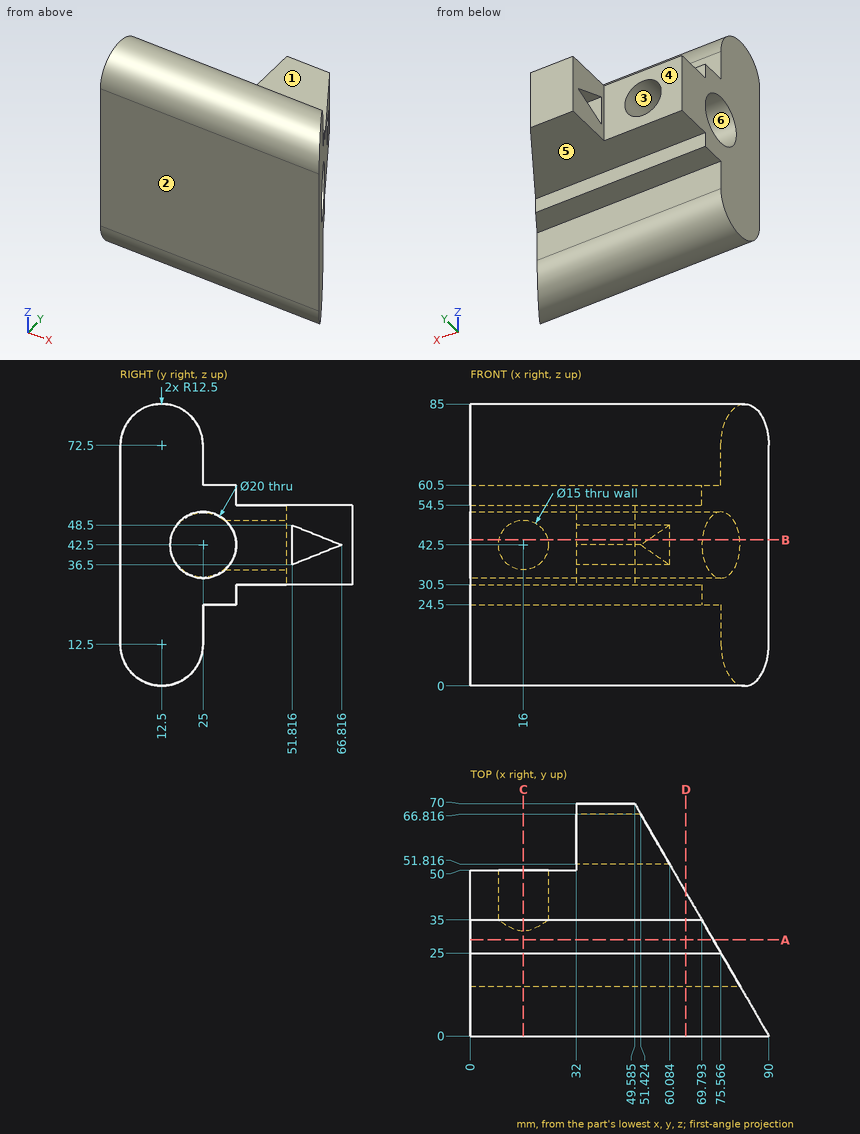
Verification items for this drawing (mm, ordinates from the low corner). A direction names the side the tool comes from. Give positions to 0.01 mm unless a question says otherwise; leave off trailing zeros. Loops run counter-clockwise (first coordinate to the right, second up) from the corner with the lowest first, then second, coordinate; pieces in that order, holes last. Notation, with made-up numbers: M 19.5,80.5 L 62.5,80.5 A20 cw 62.5,112.5 Z; hole C 36.25,74.5 d7. An arc over 180 degrees is marked long. Return JSON: item names as keys, results as strings. Group by question number.
1. Mould release check, pull along Z, two halves, no side actions. Record for the marked faces 1, 2 and 3: released by +Z, released by -Z, zero draft, split by the parting line, or undercut.
2. Cross-section at C-C on x = 16. Record the boundary of the cut face in (y, z) (1 decimal).
3. Tool access check on the marked faces 4, 5 and 6. Record the directions out of +Z, -Z, +X, -X, +Y, -Y that give a thin tool (end or side, any length) a straight path to the whole face; none if there is none.
4. Thickness scan on L1, parallel to Z at x = 16, y = 41; L2, parallel to Y at x = 33, z = 21.5; L3, parallel to X at y = 15, z = 67.5. Record the ranges inside material, lowest first.
5. Cross-section at B-B on z = 44. Record the boundary of the cut face in (x, y) (1 decimal).
6. Cross-section at D-D on x = 65. Record the boundary of the cut face in (y, z), plus the area to 3 significant figures.
7. Cross-section at A-A on y = 29. Record the boundary of the cut face in (x, z) (1 decimal).
8. Go/stop test with flat-tipped pins: pin 1 (19.5 mm diameter, centred on x = 16, z = 42.5, fed in from +Y); pin 2 (10.5 mm diameter, centred on x = 46.5, y = 60.5, fed in from +Z); pin 3 (5 mm diameter, centred on x = 31, z = 58, fed in from +Y); pin 4 (6.5 mm diameter, centred on x = 32.5, z = 27.5, fed in from +Y). Record where each tip stops, or that it passes through.
Return value:
{
 "1": {"face 1": "released by +Z", "face 2": "zero draft", "face 3": "undercut"},
 "2": {"outline": "M 0,12.5 A12.5 ccw 25,12.5 L 25,24.5 L 35,24.5 L 35,30.5 L 50,30.5 L 50,35 L 31.6,35 A10 cw long 31.6,50 L 50,50 L 50,54.5 L 35,54.5 L 35,60.5 L 25,60.5 L 25,72.5 A12.5 ccw 0,72.5 Z"},
 "3": {"face 4": "+Z, -Z, -X, +Y", "face 5": "-Z, +X, -X, +Y", "face 6": "+X, -X"},
 "4": {"L1": "30.5 to 35, 50 to 54.5", "L2": "0 to 25", "L3": "0 to 81.34"},
 "5": {"outline": "M 0,0 L 90,0 L 81.3,15.1 L 0,15.1 Z; M 0,34.9 L 8.7,34.9 L 8.7,50 L 0,50 Z; M 23.3,34.9 L 69.9,34.9 L 60.1,51.8 L 32,51.8 L 32,50 L 23.3,50 Z; M 32,63.1 L 53.6,63.1 L 49.6,70 L 32,70 Z"},
 "6": {"outline": "M 0,12.5 A12.5 ccw 25,12.5 L 25,24.5 L 35,24.5 L 35,30.5 L 43.3,30.5 L 43.3,54.5 L 35,54.5 L 35,60.5 L 25,60.5 L 25,72.5 A12.5 ccw 0,72.5 Z; hole C 25,42.5 d20", "area": "2,240 mm^2"},
 "7": {"outline": "M 0,24.5 L 73.3,24.5 L 73.3,33.3 L 0,33.3 Z; M 0,51.7 L 73.3,51.7 L 73.3,60.5 L 0,60.5 Z"},
 "8": {"pin 1": "y = 50", "pin 2": "z = 54.5", "pin 3": "y = 35", "pin 4": "y = 70"}
}
